Geometry check sheet. Reference: the model listing, model coordinates, mm. Give positions to 0.01 mm unless a question says otherwise; leave off trailing zeros. Loops run counter-clockwise (first coordinate to the right, second up) from the corner with the lowest first, then second, coordinate; pieces in that order, holes last. Notation, with made-up numbers: (34.25, -26) - (65.25, -26) arc R20 ccw to (65.25, -12) - close; hole circle Ø4 at (60, 68.25). An arc over 180 degrees is marked (long way). Write item = value, one per line. Start each with the question number.
Autodesk Inventor part; units mm, degrees
ref_plane "YZ Plane" through (0, 0, 0) normal (1, 0, 0) x (0, 1, 0)
ref_plane "XZ Plane" through (0, 0, 0) normal (0, 1, 0) x (-1, 0, 0)
ref_plane "XY Plane" through (0, 0, 0) normal (0, 0, 1) x (1, 0, 0)
sketch "Sketch1" plane through (0, 0, 0) normal (0, 0, 1) x (1, 0, 0)
  line L0 (0, 0) -> (-3.175, 0)
  line L1 (-3.175, 0) -> (-3.175, -384.175)
  line L2 (-3.175, -384.175) -> (0, -384.175)
  line L3 (0, -384.175) -> (0, 0)
  dimension "d0" = 384.175
  dimension "d1" = 3.175
extrude "Extrusion1" add sketch "Sketch1" along normal blind 152.4
chamfer "Chamfer1" distance 85.725 angle 60 1 edges at (-1.5875, -384.175, 152.4) measured on face at (-1.0583, -256.1167, 152.4)
chamfer "Chamfer2" distance 85.725 angle 60 1 edges at (-1.5875, 0, 152.4) measured on face at (-1.0583, -198.9667, 152.4)
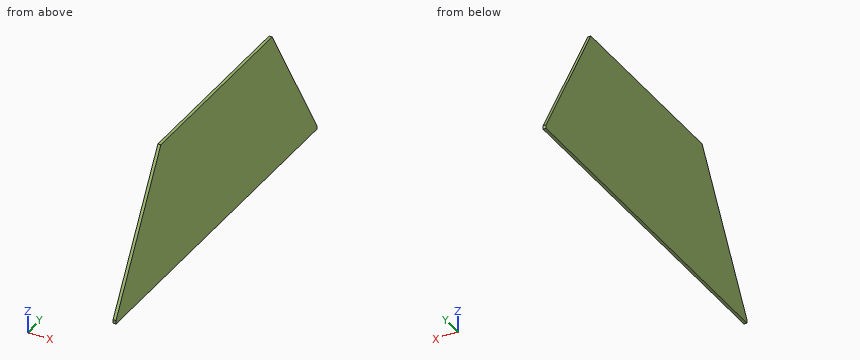
1) Cross-section at B-B on z = 101. Enter the section's corners in (x, y) (3 decimals).
2) Gauge pin test, flat end, axial feed: P1, Ø1, axis at x = -0.5, y = -303, coming from the +Z side. Record the tip position at first contact, or that the pin passes through.
3) Cross-section at C-C on y = -310. Enter the section's corners in (x, z) (3 decimals).
4) Material ranges on line 1 along Z through (x, y) = (-0.4, -299); line 2 along Y through (x, z) = (-1.05, 72.5); line 3 along Y through (x, z) = (-1.05, 33.5), recorded low to high.
5) Cross-section at A-A on x = -1.05. Enter the section's corners in (y, z) (3 decimals).
Checked values:
q1.outline = (-3.175, -328.126) - (0, -328.126) - (0, -56.049) - (-3.175, -56.049) - close
q2.P1 = 145.39
q3.outline = (-3.175, 0) - (0, 0) - (0, 132.395) - (-3.175, 132.395) - close
q4.line_1 = 0 to 151.45
q4.line_2 = -344.58 to -39.59
q4.line_3 = -367.1 to -17.08
q5.outline = (-384.175, 0) - (0, 0) - (0, 3.92) - (-85.725, 152.4) - (-298.45, 152.4) - (-384.175, 3.92) - close
